Design review of the part built by this model. Coordinates are the model's own, in mm. Face numbers are marked on the shaded views. A direction names the side the tool comes from. Round coordinates to 2 decimals unless told otherwise and drop trailing zeros. Write each loop counter-clockwise with the first axis right and the second up, starting at its lowest first coordinate (ties: lowest second). Pieces come first, ordered by that corner, then holes. Notation, with made-up numbers: (83.25, 16.25) -> (98.25, 16.25) arc R25 cw to (98.25, 45.25) -> close; hole circle Ø10 at (-28.75, 6). An arc over 180 degrees is marked (long way). One line per question, with ' | ' between items. Start each with the question number.
1) Consider section A-A (y = 19). Give the boundary of the cut face in (x, z), then the cut area to 3 significant figures.
2) Consider section B-B (x = 68.5). Give the boundary of the cut face in (y, z), then the cut area to 3 significant figures.
3) For probe 1 along Z at (x, y) = (10.5, 7.25); probe 2 along Z at (x, y) = (49.6, 6); probe 3 along Y at (x, z) = (25, 78.65), list the stretches that pass through material, from the lowest coordinate up.
4) Mouldability with a two-part tool opening along X and no side actions: class the marked faces 1, 2 and 3 as +X half, -X half, draft (parallel to the pull), parting line (faces both ways), or undercut.
5) For the marked faces 4, 5 and 6, list the 3-axis set-ups (+Z, -Z, +X, -X, +Y, -Y) from which the entire face can be reached by the end or side of a thin tool; tool diameter is ignored.
6) Insertion check: pin 1 Ø3 at (y, z) = (13.5, 41.5) entering from +X; pin 2 Ø10 at (x, z) = (61, -12.5) entering from +Y; pin 3 Ø10 at (x, y) = (63.5, 4) entering from +Z. Each pin has a flat end and moves straight along its axis. Give the tip position at first contact, or say it passes through.
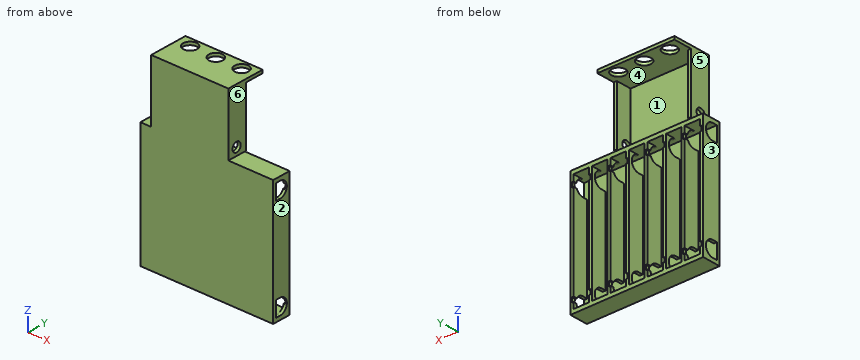
```python
from build123d import *

# Parameters (mm, degrees)
SKETCH1_W               = 14
SKETCH1_H               = 80
BOSS_EXTRUDE1_DEPTH     = 2
SKETCH2_W               = 14
SKETCH2_H               = 80
SKETCH2_W_2             = 10
SKETCH2_H_2             = 75
BOSS_EXTRUDE2_DEPTH     = 10
SKETCH3_W               = 1
SKETCH3_H               = 3
CUT_EXTRUDE1_DEPTH      = 10
CUT_EXTRUDE2_DEPTH      = 14
SKETCH5_W               = 72
SKETCH5_H               = 80
BOSS_EXTRUDE3_DEPTH     = 2
SKETCH6_W               = 14
SKETCH6_H               = 80
SKETCH6_W_2             = 10
SKETCH6_H_2             = 75
BOSS_EXTRUDE4_DEPTH     = 10
MIRROR2_COPY_1_SKETCH_W = 1
MIRROR2_COPY_1_SKETCH_H = 3
MIRROR2_COPY_1_DEPTH    = 10
MIRROR5_COPY_1_DEPTH    = 14
SKETCH7_W               = 10
SKETCH7_H               = 2.5
BOSS_EXTRUDE5_DEPTH     = 10
SKETCH8_W               = 50
SKETCH8_H               = 40
BOSS_EXTRUDE6_DEPTH     = 3
BOSS_EXTRUDE7_DEPTH     = 10
SKETCH10_R              = 3
CUT_EXTRUDE3_DEPTH      = 50
SKETCH11_W              = 50
SKETCH11_H              = 2
BOSS_EXTRUDE8_DEPTH     = 12
SKETCH12_R              = 4.5
CUT_EXTRUDE4_DEPTH      = 2


with BuildPart() as part:
    # Sketch1 → Boss-Extrude1 (new body)
    with BuildSketch(Plane(origin=(0, 0, 0), x_dir=(1, 0, 0), z_dir=(0, 1, 0))):
        Rectangle(SKETCH1_W, SKETCH1_H)
    extrude(amount=BOSS_EXTRUDE1_DEPTH)

    # Sketch2 → Boss-Extrude2 (add)
    with BuildSketch(Plane(origin=(0, 2, 0), x_dir=(1, 0, 0), z_dir=(0, 1, 0))):
        Rectangle(SKETCH2_W, SKETCH2_H)
        Rectangle(SKETCH2_W_2, SKETCH2_H_2, mode=Mode.SUBTRACT)
    extrude(amount=BOSS_EXTRUDE2_DEPTH)

    # Sketch3 → Cut-Extrude1 (cut)
    with BuildSketch(Plane(origin=(0, 12, 0), x_dir=(1, 0, 0), z_dir=(0, 1, 0))):
        with Locations((-5.5, -32)):
            Rectangle(SKETCH3_W, SKETCH3_H)
        with Locations((5.5, -32)):
            Rectangle(SKETCH3_W, SKETCH3_H)
        with Locations((5.5, 32)):
            Rectangle(SKETCH3_W, SKETCH3_H)
        with Locations((-5.5, 32)):
            Rectangle(SKETCH3_W, SKETCH3_H)
    cut_extrude1 = extrude(amount=-CUT_EXTRUDE1_DEPTH, mode=Mode.SUBTRACT)

    # Sketch4 → Cut-Extrude2 (cut)
    with BuildSketch(Plane(origin=(7, 0, 0), x_dir=(0, 0, -1), z_dir=(1, 0, 0))):
        with BuildLine():
            ThreePointArc((-37.5, 5), (-32.5, 10), (-27.5, 5))
            Line((-27.5, 5), (-27.5, 2))
            Line((-27.5, 2), (-32.5, 2))
            Line((-32.5, 2), (-37.5, 2))
            Line((-37.5, 2), (-37.5, 5))
        make_face()
        with BuildLine():
            ThreePointArc((27.5, 5), (32.5, 10), (37.5, 5))
            Line((37.5, 5), (37.5, 2))
            Line((37.5, 2), (32.5, 2))
            Line((32.5, 2), (27.5, 2))
            Line((27.5, 2), (27.5, 5))
        make_face()
    cut_extrude2 = extrude(amount=-CUT_EXTRUDE2_DEPTH, mode=Mode.SUBTRACT)

    # Sketch5 → Boss-Extrude3 (add)
    with BuildSketch(Plane(origin=(0, 0, 0), x_dir=(1, 0, 0), z_dir=(0, 1, 0))):
        with Locations((43, 0)):
            Rectangle(SKETCH5_W, SKETCH5_H)
    extrude(amount=BOSS_EXTRUDE3_DEPTH)

    # Sketch6 → Boss-Extrude4 (add)
    # profile 1 of 3: a face of its own
    with BuildSketch(Plane(origin=(0, 2, 0), x_dir=(1, 0, 0), z_dir=(0, 1, 0))):
        with Locations((24, 0)):
            Rectangle(SKETCH6_W, SKETCH6_H)
        with Locations((24, 0)):
            Rectangle(SKETCH6_W_2, SKETCH6_H_2, mode=Mode.SUBTRACT)
    # profile 2 of 3: a face of its own
    with BuildSketch(Plane(origin=(0, 2, 0), x_dir=(1, 0, 0), z_dir=(0, 1, 0))):
        with Locations((48, 0)):
            Rectangle(SKETCH6_W, SKETCH6_H)
        with Locations((48, 0)):
            Rectangle(SKETCH6_W_2, SKETCH6_H_2, mode=Mode.SUBTRACT)
    # profile 3 of 3: a face of its own
    with BuildSketch(Plane(origin=(0, 2, 0), x_dir=(1, 0, 0), z_dir=(0, 1, 0))):
        with Locations((72, 0)):
            Rectangle(SKETCH6_W, SKETCH6_H)
        with Locations((72, 0)):
            Rectangle(SKETCH6_W_2, SKETCH6_H_2, mode=Mode.SUBTRACT)
    extrude(amount=BOSS_EXTRUDE4_DEPTH)

    # Mirror1: Cut-Extrude1 across plane
    add(cut_extrude1.mirror(Plane.ZY.offset(-12)), mode=Mode.SUBTRACT)

    # Mirror2: Cut-Extrude1 across plane
    add(cut_extrude1.mirror(Plane.ZY.offset(-36)), mode=Mode.SUBTRACT)

    # Mirror2 copy 1 sketch → Mirror2 copy 1 (cut)
    with BuildSketch(Plane(origin=(48, 12, 0), x_dir=(1, 0, 0), z_dir=(0, 1, 0))):
        with Locations((-5.5, -32)):
            Rectangle(MIRROR2_COPY_1_SKETCH_W, MIRROR2_COPY_1_SKETCH_H)
        with Locations((5.5, -32)):
            Rectangle(MIRROR2_COPY_1_SKETCH_W, MIRROR2_COPY_1_SKETCH_H)
        with Locations((5.5, 32)):
            Rectangle(MIRROR2_COPY_1_SKETCH_W, MIRROR2_COPY_1_SKETCH_H)
        with Locations((-5.5, 32)):
            Rectangle(MIRROR2_COPY_1_SKETCH_W, MIRROR2_COPY_1_SKETCH_H)
    extrude(amount=-MIRROR2_COPY_1_DEPTH, mode=Mode.SUBTRACT)

    # Mirror4: Cut-Extrude2 across plane
    add(cut_extrude2.mirror(Plane.ZY.offset(-12)), mode=Mode.SUBTRACT)

    # Mirror5: Cut-Extrude2 across plane
    add(cut_extrude2.mirror(Plane.ZY.offset(-36)), mode=Mode.SUBTRACT)

    # Mirror5 copy 1 sketch → Mirror5 copy 1 (cut)
    with BuildSketch(Plane(origin=(55, 0, 0), x_dir=(0, 0, -1), z_dir=(1, 0, 0))):
        with BuildLine():
            ThreePointArc((-37.5, 5), (-32.5, 10), (-27.5, 5))
            Line((-27.5, 5), (-27.5, 2))
            Line((-27.5, 2), (-32.5, 2))
            Line((-32.5, 2), (-37.5, 2))
            Line((-37.5, 2), (-37.5, 5))
        make_face()
        with BuildLine():
            ThreePointArc((27.5, 5), (32.5, 10), (37.5, 5))
            Line((37.5, 5), (37.5, 2))
            Line((37.5, 2), (32.5, 2))
            Line((32.5, 2), (27.5, 2))
            Line((27.5, 2), (27.5, 5))
        make_face()
    extrude(amount=-MIRROR5_COPY_1_DEPTH, mode=Mode.SUBTRACT)

    # Sketch7 → Boss-Extrude5 (add)
    with BuildSketch(Plane(origin=(0, 2, 0), x_dir=(1, 0, 0), z_dir=(0, 1, 0))):
        with Locations((12, 38.75)):
            Rectangle(SKETCH7_W, SKETCH7_H)
        with Locations((36, 38.75)):
            Rectangle(SKETCH7_W, SKETCH7_H)
        with Locations((60, 38.75)):
            Rectangle(SKETCH7_W, SKETCH7_H)
        with Locations((60, -38.75)):
            Rectangle(SKETCH7_W, SKETCH7_H)
        with Locations((36, -38.75)):
            Rectangle(SKETCH7_W, SKETCH7_H)
        with Locations((12, -38.75)):
            Rectangle(SKETCH7_W, SKETCH7_H)
    extrude(amount=BOSS_EXTRUDE5_DEPTH)

    # Sketch8 → Boss-Extrude6 (add)
    with BuildSketch(Plane(origin=(0, 0, 0), x_dir=(1, 0, 0), z_dir=(0, 1, 0))):
        with Locations((25, -60)):
            Rectangle(SKETCH8_W, SKETCH8_H)
    extrude(amount=BOSS_EXTRUDE6_DEPTH)

    # Sketch9 → Boss-Extrude7 (add)
    with BuildSketch(Plane(origin=(0, 3, 0), x_dir=(1, 0, 0), z_dir=(0, 1, 0))):
        Polygon((0, -40), (0, -80), (50, -80), (50, -40), (48, -40), (48, -78), (2, -78), (2, -40), align=None)
    extrude(amount=BOSS_EXTRUDE7_DEPTH)

    # Sketch10 → Cut-Extrude3 (cut)
    with BuildSketch(Plane.ZY):
        with Locations((45, 6)):
            Circle(SKETCH10_R)
    extrude(amount=-CUT_EXTRUDE3_DEPTH, mode=Mode.SUBTRACT)

    # Sketch11 → Boss-Extrude8 (add)
    with BuildSketch(Plane(origin=(0, 13, 0), x_dir=(1, 0, 0), z_dir=(0, 1, 0))):
        with Locations((25, -79)):
            Rectangle(SKETCH11_W, SKETCH11_H)
    extrude(amount=BOSS_EXTRUDE8_DEPTH)

    # Sketch12 → Cut-Extrude4 (cut)
    with BuildSketch(Plane.XY.offset(80)):
        with Locations((8.333333333, 19)):
            Circle(SKETCH12_R)
        with Locations((25, 19)):
            Circle(SKETCH12_R)
        with Locations((41.666666667, 19)):
            Circle(SKETCH12_R)
    extrude(amount=-CUT_EXTRUDE4_DEPTH, mode=Mode.SUBTRACT)


solid = part.part
```
From the geometry:
1) outline: (0, 78) -> (3.83, 78) -> (3.83, 80) -> (0, 80) -> close; (12.83, 78) -> (20.5, 78) -> (20.5, 80) -> (12.83, 80) -> close; (29.5, 78) -> (37.17, 78) -> (37.17, 80) -> (29.5, 80) -> close; (46.17, 78) -> (50, 78) -> (50, 80) -> (46.17, 80) -> close | area: 46.0 mm2
2) outline: (0, -40) -> (12, -40) -> (12, -37.5) -> (2, -37.5) -> (2, 37.5) -> (12, 37.5) -> (12, 40) -> (0, 40) -> close | area: 210 mm2
3) probe 1: z = -40 to -37.5, 37.5 to 40, 78 to 80 | probe 2: z = -40 to -37.5, 37.5 to 42, 48 to 80 | probe 3: y = 0 to 14.5, 23.5 to 25
4) face 1: undercut | face 2: +X half | face 3: -X half
5) face 4: +Y | face 5: +Z, -X, +Y, -Y | face 6: +Z, +X, +Y, -Y
6) pin 1: stops at x = 50 | pin 2: stops at y = 12 | pin 3: stops at z = 40
